from build123d import *

# Parameters (mm, degrees)
F0_W            = 42.8076982498
F0_H            = 5
F1_DEPTH        = 34
F2_R            = 5
F3_R            = 5
F4_R            = 5
F5_R            = 5
F6_R            = 5
F7_R            = 5
F10_D           = 3
F10_CSINK_D     = 4
F10_CSINK_ANGLE = 90
F11_D           = 3
F11_CSINK_D     = 4
F11_CSINK_ANGLE = 90


with BuildPart() as f1:
    # F0 (on Front) → F1 (new body)
    with BuildSketch(Plane.XZ):
        Polygon((-30.423078686, 35.2884634584), (-37.9615426064, 35.2884634584), (-37.9615426064, -29.8653867841), (-30.423078686, -29.8653867841), (-30.423078686, -24.8653867841), (-30.423078686, 30.2884634584), align=None)
        with Locations((-9.0192295611, 32.7884634584)):
            Rectangle(F0_W, F0_H)
        with Locations((-9.0192295611, -27.3653867841)):
            Rectangle(F0_W, F0_H)
    extrude(amount=F1_DEPTH)

    # F2
    f2_edges = [f1.edges().sort_by_distance(p)[0] for p in [
        (12.38462, -34, 32.788463),
    ]]
    fillet(f2_edges, radius=F2_R)

    # F3
    f3_edges = [f1.edges().sort_by_distance(p)[0] for p in [
        (12.38462, 0, 32.788463),
    ]]
    fillet(f3_edges, radius=F3_R)

    # F4
    f4_edges = [f1.edges().sort_by_distance(p)[0] for p in [
        (12.38462, -34, -27.365387),
    ]]
    fillet(f4_edges, radius=F4_R)

    # F5
    f5_edges = [f1.edges().sort_by_distance(p)[0] for p in [
        (12.38462, 0, -27.365387),
    ]]
    fillet(f5_edges, radius=F5_R)

    # F6
    f6_edges = [f1.edges().sort_by_distance(p)[0] for p in [
        (-37.961543, -17, 35.288463),
    ]]
    fillet(f6_edges, radius=F6_R)

    # F7
    f7_edges = [f1.edges().sort_by_distance(p)[0] for p in [
        (-30.423079, -17, -24.865387),
        (-30.423079, -17, 30.288463),
        (-37.961543, -17, -29.865387),
    ]]
    fillet(f7_edges, radius=F7_R)

    # F10 (through all)
    with Locations(Plane(origin=(-37.9615426064, 0, 0), x_dir=(0, -1, 0), z_dir=(-1, 0, 0))):
        with Locations((12.5500056893, 0), (20.5500056893, 0), (28.5500056893, 0)):
            CounterSinkHole(F10_D / 2, F10_CSINK_D / 2, counter_sink_angle=F10_CSINK_ANGLE)

    # F11 (through all)
    with Locations(Plane.XY.offset(35.2884634584)):
        with Locations((-0.3527658135, -16.5143854618), (-8.3527658135, -16.5143854618), (7.6472341865, -16.5143854618)):
            CounterSinkHole(F11_D / 2, F11_CSINK_D / 2, counter_sink_angle=F11_CSINK_ANGLE)


solid = f1.part
Can you work these out from the model? Positions are in its coordinate system, mm. A direction names the side the tool comes from. Give positions to 0.01 mm unless a question says otherwise; leave off trailing zeros. Order: outer loops, then holes, each group sorted by start corner. A loop starts at its lowest first (then second) coordinate and runs counter-clockwise, first axis right, second up. Notation, with made-up numbers: M -22.75,-8 L -7.75,-8 A29 cw -7.75,14 Z; hole C 86.5,23 d5. An arc over 180 degrees is marked long. One line per question, with ' | ' between items.
Item 1: Suppose I cut it at A-A, the plane x = -16. Write out the boundary of the cut face in (y, z), then the cut area to 3 significant figures.
Answer block:
outline: M -34,-29.87 L 0,-29.87 L 0,-24.87 L -34,-24.87 Z; M -34,30.29 L 0,30.29 L 0,35.29 L -34,35.29 Z | area: 340 mm2
Item 2: We'd pull the mould along Z, two halves only. Please class faces 1 (the face through (-37.962, -17, 3)), 2 (the face through (-36.54, -17.24, 33.78)), 3 (the face through (-7, -13, 30.288)): released by +Z, released by -Z, zero draft, split by the parting line, or undercut.
Answer block:
face 1: zero draft | face 2: released by +Z | face 3: undercut
Item 3: Suppose I cut it at C-C, the plane x = -27.5. Write out the boundary of the cut face in (y, z).
Answer block:
outline: M -34,-29.87 L 0,-29.87 L 0,-24.41 L -34,-24.41 Z; M -34,29.84 L 0,29.84 L 0,35.29 L -34,35.29 Z
Item 4: I'm going to push flat-ended pins straight in: pin 1 Ø2.5 at (y, z) = (-20.55, 0) entering from -X; pin 2 Ø3.5 at (x, y) = (-8.35, -16.51) entering from +Z; pin 3 Ø10 at (x, z) = (-28.5, 2) entering from +Y; pin 4 Ø3.5 at (y, z) = (-12.55, 0) entering from -X. Where does each tip first touch, or does it pass through?
Answer block:
pin 1: passes through | pin 2: stops at z = 35.04 | pin 3: stops at y = 0 | pin 4: stops at x = -37.71
Item 5: Suppose I cut it at B-B, the plane z = 0. Write out the boundary of the cut face in (x, y), then the cut area to 3 significant figures.
Answer block:
outline: M -37.96,-34 L -30.42,-34 L -30.42,-30.05 L -37.46,-30.05 L -37.96,-30.55 Z; M -37.96,-26.55 L -37.46,-27.05 L -30.42,-27.05 L -30.42,-22.05 L -37.46,-22.05 L -37.96,-22.55 Z; M -37.96,-18.55 L -37.46,-19.05 L -30.42,-19.05 L -30.42,-14.05 L -37.46,-14.05 L -37.96,-14.55 Z; M -37.96,-10.55 L -37.46,-11.05 L -30.42,-11.05 L -30.42,0 L -37.96,0 Z | area: 188 mm2
Item 6: For faces 4 (the face through (-28.92, -17.24, 28.86)), 5 (the face through (-9.16, -15.25, -27.4)), which set-ups out of +Z, -Z, +X, -X, +Y, -Y let a thin tool reach every point of the face, with its end or its side?
Answer block:
face 4: +X, +Y, -Y | face 5: +Z, -Z
Item 7: Please list where these lines run through material, in increasing order: L1, parallel to Z at x = -11, y = -24; L2, parallel to X at y = -18, z = 4; L3, parallel to Z at x = -28.5, y = -31.
Answer block:
L1: z = -29.87 to -24.87, 30.29 to 35.29 | L2: x = -37.96 to -30.42 | L3: z = -29.87 to -23.81, 29.23 to 35.29
